Read the model definition and answer for the solid it produces. Units are mm, in the model's axes. A direction names the side the tool comes from. Coordinates: 2 decimals unless noted, no trailing zeros. Order: outer loops, then holes, each group sorted by start corner. A loop starts at its lowest first (then second) coordinate and runs counter-clockwise, first axis right, second up. Notation, with made-up numbers: (61, 16) - (105, 16) arc R26 cw to (105, 33) - close; hole circle Ø1 at (28.5, 34.5). An arc over 180 degrees is marked (long way). Use one line per item in the form item = value. Start each with the question number.
from build123d import *

# Parameters (mm, degrees)
ESQUISSE1_W             = 40
ESQUISSE1_H             = 30
BOSS_EXTRU_1_DEPTH      = 5
ESQUISSE2_W             = 40
ESQUISSE2_H             = 5
BOSS_EXTRU_2_DEPTH      = 10
ESQUISSE3_R             = 1.625
ENL_V_MAT_EXTRU_1_DEPTH = 6
ESQUISSE4_R             = 2.6
ENL_V_MAT_EXTRU_2_DEPTH = 4


with BuildPart() as part:
    # Esquisse1 → Boss.-Extru.1 (new body)
    with BuildSketch(Plane.XY):
        with Locations((20, -15)):
            Rectangle(ESQUISSE1_W, ESQUISSE1_H)
    extrude(amount=BOSS_EXTRU_1_DEPTH)

    # Esquisse2 → Boss.-Extru.2 (add)
    with BuildSketch(Plane.XY.offset(5)):
        with Locations((20, -2.5)):
            Rectangle(ESQUISSE2_W, ESQUISSE2_H)
    extrude(amount=BOSS_EXTRU_2_DEPTH)

    # Esquisse3 → Enlèv. mat.-Extru.1 (cut, through all)
    with BuildSketch(Plane.XZ.offset(5)):
        with Locations((5, 10)):
            Circle(ESQUISSE3_R)
        with Locations((35, 10)):
            Circle(ESQUISSE3_R)
    extrude(amount=-ENL_V_MAT_EXTRU_1_DEPTH, mode=Mode.SUBTRACT)

    # Esquisse4 → Enlèv. mat.-Extru.2 (cut)
    with BuildSketch(Plane(origin=(0, 0, 0), x_dir=(-1, 0, 0), z_dir=(0, 0, -1))):
        with Locations((-9.1, -20.9)):
            Circle(ESQUISSE4_R)
    extrude(amount=-ENL_V_MAT_EXTRU_2_DEPTH, mode=Mode.SUBTRACT)


solid = part.part
Q1. A cutting plane is placed at B-B (x = 5). Give the vertices of the cut face in (y, z) (3 decimals), then the cut area to 3 significant figures.
Q2. A cutting plane is placed at A-A (z = 10). Give the vertices of the cut face in (x, y) (3 decimals), then the cut area to 4 significant figures.
Q3. Which of the six approach directions +Z, -Z, +X, -X, +Y, -Y give full straight-line access (tool end or side, diameter ignored) to faces 1 (the flat face through (20, -2, 15)), 2 (the flat face through (9, -21, 4)), 3 (the flat face through (20, -5, 10))?
Q4. Consider probe 1 along Z at (x, y) = (35, -1.25) (3 decimals); probe 2 along Z at (x, y) = (5, -24.75); probe 3 along Y at (x, z) = (26, 9.75). Determine where each line is inside the solid, lowest interval first.
Q5. A cutting plane is placed at C-C (y = -20.9). Give the vertices of the cut face in (x, z).
Q6. For a pull along Y with two mould halves and no side action, classify faces 4 (the cylindrical face through (6.62, -20.12, 1.97)), 5 (the flat face through (20, 0, 7)), 6 (the flat face through (20, -15, 0)) as +Y half, -Y half, draft (parallel to the pull), parting line (faces both ways), or undercut.
Q7. A cutting plane is placed at D-D (x = 9.1). Give the vertices of the cut face in (y, z), then the cut area to 3 significant figures.
Q8. Given P1, Ø8, axis at x = 20.5, y = -21.5, coming from the +Z side; P2, Ø2.5, axis at x = 8, y = -21, coming from the -Z side; P3, Ø1.9, axis at x = 35, z = 10, coming from the -Y side; P4, Ø4, axis at x = 28.5, y = -4, coming from the -Z side, each flat-ended and moving along its own axis, determine where each tip first touches the part or whether it passes through.
Result sheet:
q1.outline = (-30, 0) - (0, 0) - (0, 8.375) - (-5, 8.375) - (-5, 5) - (-30, 5) - close; (-5, 11.625) - (0, 11.625) - (0, 15) - (-5, 15) - close
q1.area = 184 mm^2
q2.outline = (0, -5) - (3.375, -5) - (3.375, 0) - (0, 0) - close; (6.625, -5) - (33.375, -5) - (33.375, 0) - (6.625, 0) - close; (36.625, -5) - (40, -5) - (40, 0) - (36.625, 0) - close
q2.area = 167.5 mm^2
q3.face_1 = +Z, +X, -X, +Y, -Y
q3.face_2 = -Z
q3.face_3 = +Z, +X, -X, -Y
q4.probe_1 = 0 to 8.375, 11.625 to 15
q4.probe_2 = 0 to 5
q4.probe_3 = -5 to 0
q5.outline = (0, 0) - (6.5, 0) - (6.5, 4) - (11.7, 4) - (11.7, 0) - (40, 0) - (40, 5) - (0, 5) - close
q6.face_4 = undercut
q6.face_5 = +Y half
q6.face_6 = draft
q7.outline = (-30, 0) - (-23.5, 0) - (-23.5, 4) - (-18.3, 4) - (-18.3, 0) - (0, 0) - (0, 15) - (-5, 15) - (-5, 5) - (-30, 5) - close
q7.area = 179 mm^2
q8.P1 = 5
q8.P2 = 4
q8.P3 = through
q8.P4 = 0
